```python
from build123d import *


with BuildPart() as part:
    # Esquisse1 → R_volution1 (revolve)
    with BuildSketch(Plane.XY, mode=Mode.PRIVATE) as r_volution1_sk:
        with BuildLine():
            Line((-1.36, 44.5), (0, 44.5))
            Line((0, 44.5), (0, 0))
            Line((0, 0), (-4.95, 0))
            ThreePointArc((-4.95, 0), (-5.162132034, 0.087867966), (-5.25, 0.3))
            Line((-5.25, 0.3), (-5.25, 41.926794919))
            ThreePointArc((-5.25, 41.926794919), (-5.232962913, 42.056204442), (-5.183012702, 42.176794919))
            Line((-5.183012702, 42.176794919), (-4.65, 43.1))
            ThreePointArc((-4.65, 43.1), (-4.576794919, 43.173205081), (-4.476794919, 43.2))
            Line((-4.476794919, 43.2), (-3.5, 43.2))
            Line((-3.5, 43.2), (-3.5, 43))
            Line((-3.5, 43), (-1.86, 43))
            Line((-1.86, 43), (-1.86, 44))
            ThreePointArc((-1.86, 44), (-1.713553391, 44.353553391), (-1.36, 44.5))
        make_face()
    revolve(r_volution1_sk.sketch.rotate(Axis((0, 0, 0), (0, 1, 0)), 270), axis=Axis((0, 0, 0), (0, 1, 0)))


solid = part.part
```
Read the model definition and answer for the solid it produces. Units are mm, in the model's axes. A direction names the side the tool comes from. Give positions to 0.01 mm unless a question says otherwise; leave off trailing zeros. Order: outer loops, then holes, each group sorted by start corner. A loop starts at its lowest first (then second) coordinate and runs counter-clockwise, first axis right, second up. Notation, with made-up numbers: (14.5, -11) -> (72.5, -11) arc R32 ccw to (72.5, 24) -> close; hole circle Ø7 at (45.25, -4.5). An arc over 180 degrees is marked (long way). One line per item, written item: value. Start each with the question number.
(1) Straight lines are drawn through the part: L1, parallel to X at y = 43.15, z = 0; L2, parallel to X at y = 43.05, z = 0; L3, parallel to X at y = 40.5, z = -1.75. For each, find the intervals that lie inside material, in ascending order.
(2) For a pull along X with two mould halves and no side action, classify faces 3 (the cylindrical face through (-1.6, 21.4, -5)), 4 (the flat face through (2, 43, -2)), 5 (the flat face through (4, 43.2, 0)) as released by +X, released by -X, zero draft, split by the parting line, or undercut.
(3) The part is cut by section A-A (x = 0). Determine the outline of the cut face in (y, z), and give its area (3 significant figures).
(4) Flat-ended cylindrical pins translate along their axes: P1, Ø3, axis at x = -4, z = 0, coming from the +Y side; P2, Ø1.5, axis at x = 2, y = 18.5, coming from the -Z side. Find the tip coordinate at first contact, or state that the pin passes through.
(5) The part is cut by section C-C (y = 20). Determine the outline of the cut face in (x, z), and give its area (3 significant figures).
(6) The part is cut by section B-B (z = 0). Determine the outline of the cut face in (x, y), and give its area (3 significant figures).
(7) A tool of negligible diameter and unlimited length cuts with its end or side. For faces 1 (the flat face through (0, 44.5, 0)), 2 (the cylindrical face through (-0.08, 43.51, 1.86)), from which of +Z, -Z, +X, -X, +Y, -Y can it reach the whole face along a straight path? Write none if from no direction.
Taken from the geometry:
1. L1: -4.61 to -3.5, -1.86 to 1.86, 3.5 to 4.61
1. L2: -4.68 to -3.5, -1.86 to 1.86, 3.5 to 4.68
1. L3: -4.95 to 4.95
2. face 3: split by the parting line
2. face 4: undercut
2. face 5: zero draft
3. outline: (0, -4.95) arc R0.3 ccw to (0.3, -5.25) -> (41.93, -5.25) arc R0.5 ccw to (42.18, -5.18) -> (43.1, -4.65) arc R0.2 ccw to (43.2, -4.48) -> (43.2, -3.5) -> (43, -3.5) -> (43, -1.86) -> (44, -1.86) arc R0.5 ccw to (44.5, -1.36) -> (44.5, 1.36) arc R0.5 ccw to (44, 1.86) -> (43, 1.86) -> (43, 3.5) -> (43.2, 3.5) -> (43.2, 4.48) arc R0.2 ccw to (43.1, 4.65) -> (42.18, 5.18) arc R0.5 ccw to (41.93, 5.25) -> (0.3, 5.25) arc R0.3 ccw to (0, 4.95) -> close
3. area: 457 mm^2
4. P1: y = 43.2
4. P2: z = -5.1
5. outline: circle Ø10.5 at (0, 0)
5. area: 86.6 mm^2
6. outline: (-5.25, 0.3) arc R0.3 ccw to (-4.95, 0) -> (4.95, 0) arc R0.3 ccw to (5.25, 0.3) -> (5.25, 41.93) arc R0.5 ccw to (5.18, 42.18) -> (4.65, 43.1) arc R0.2 ccw to (4.48, 43.2) -> (3.5, 43.2) -> (3.5, 43) -> (1.86, 43) -> (1.86, 44) arc R0.5 ccw to (1.36, 44.5) -> (-1.36, 44.5) arc R0.5 ccw to (-1.86, 44) -> (-1.86, 43) -> (-3.5, 43) -> (-3.5, 43.2) -> (-4.48, 43.2) arc R0.2 ccw to (-4.65, 43.1) -> (-5.18, 42.18) arc R0.5 ccw to (-5.25, 41.93) -> close
6. area: 457 mm^2
7. face 1: +Z, -Z, +X, -X, +Y
7. face 2: +Y
